```python
from build123d import *

# Parameters (mm, degrees)
F0_W     = 23.7
F0_H     = 15.8
F1_DEPTH = 10
F2_R     = 2.75
F3_DEPTH = 3
F4_W     = 20.786194
F4_H     = 12.840617
F5_DEPTH = 8
F6_R     = 3.802905
F6_R_2   = 2.49672
F6_R_3   = 2.479142
F7_DEPTH = 8


with BuildPart() as f1:
    # F0 (on Top) → F1 (new body)
    with BuildSketch(Plane.XY):
        with Locations((11.85, 7.9)):
            Rectangle(F0_W, F0_H)
    extrude(amount=F1_DEPTH)

    # F2 (on face) → F3 (join)
    with BuildSketch(Plane.XY.offset(10)):
        with Locations((4.25, 11.85)):
            Circle(F2_R)
        with Locations((11.75, 11.85)):
            Circle(F2_R)
        with Locations((19.25, 11.85)):
            Circle(F2_R)
        with Locations((4.25, 4.115675)):
            Circle(F2_R)
        with Locations((11.75, 4.115675)):
            Circle(F2_R)
        with Locations((19.25, 4.115675)):
            Circle(F2_R)
    extrude(amount=F3_DEPTH)

    # F4 (on face) → F5 (cut)
    with BuildSketch(Plane(origin=(0, 0, 0), x_dir=(1, 0, 0), z_dir=(0, 0, -1))):
        with Locations((11.888078, -7.852494)):
            Rectangle(F4_W, F4_H)
    extrude(amount=-F5_DEPTH, mode=Mode.SUBTRACT)

    # F6 (on face) → F7 (join)
    with BuildSketch(Plane(origin=(0, 0, 8), x_dir=(1, 0, 0), z_dir=(0, 0, -1))):
        with Locations((16.33504, -7.714347)):
            Circle(F6_R)
        with Locations((16.33504, -7.714347)):
            Circle(F6_R_2, mode=Mode.SUBTRACT)
        with Locations((6.87801, -7.714347)):
            Circle(F6_R)
        with Locations((6.87801, -7.714347)):
            Circle(F6_R_3, mode=Mode.SUBTRACT)
    extrude(amount=F7_DEPTH)


solid = f1.part
```
Here's how the part is built. I have some questions about the finished solid (model axes, mm). A direction names the side the tool comes from. Coordinates: 2 decimals unless noted, no trailing zeros. Order: outer loops, then holes, each group sorted by start corner. A loop starts at its lowest first (then second) coordinate and runs counter-clockwise, first axis right, second up. Notation, with made-up numbers: (-26, 18) - (22, 18) arc R35 cw to (22, 52) - close; hole circle Ø1 at (12, 30). An arc over 180 degrees is marked (long way). One line per question, with ' | ' between items. Start each with the question number.
1. If we section it at D-D (z = 10.75): Write out the boundary of the cut face in (x, y).
2. If we section it at A-A (z = 6.5): Write out the boundary of the cut face in (x, y).
3. Please list where these lines run through material, in increasing order: line 1 along Y through (x, z) = (4, 5.5); line 2 along Y through (x, z) = (11.25, 3.5); line 3 along X through (y, z) = (8, 1.5). Write a range as [from, to].
4. If we mould it in two halves opening along Y, with no side actions, what happens to faces 1 (the flat face through (19, 9, 0)), 2 (the cylindrical face through (18.09, 11.09, 4.06)), 3 (the flat face through (12, 15.8, 5))? For each: released by +Y, released by -Y, zero draft, split by the parting line, or undercut.
5. Which directions (+Z, -Z, +X, -X, +Y, -Y) give clear straight access to the entire face, cutting with the end or side of a thin tool? Please do faces 4 (the flat face through (4, 12, 13)), 5 (the cylindrical face through (5.5, 9.4, 11.5)), 6 (the cylindrical face through (13.84, 7.6, 4.06)).
6. If we section it at C-C (x = 11.75): Write out the boundary of the cut face in (y, z).
7. If we section it at B-B (y = 11.85): Write out the boundary of the cut face in (x, z).
Model answer:
1) outline: circle Ø5.5 at (4.25, 4.12); circle Ø5.5 at (4.25, 11.85); circle Ø5.5 at (11.75, 4.12); circle Ø5.5 at (11.75, 11.85); circle Ø5.5 at (19.25, 4.12); circle Ø5.5 at (19.25, 11.85)
2) outline: (0, 0) - (23.7, 0) - (23.7, 15.8) - (0, 15.8) - close; circle Ø7.61 at (6.88, 7.71); circle Ø7.61 at (16.34, 7.71); hole (1.49, 1.43) - (22.28, 1.43) - (22.28, 14.27) - (1.49, 14.27) - close; hole circle Ø4.96 at (6.88, 7.71); hole circle Ø4.99 at (16.34, 7.71)
3) line 1: y = [0, 1.43], [5.23, 10.2], [14.27, 15.8] | line 2: y = [0, 1.43], [14.27, 15.8] | line 3: x = [0, 1.49], [3.09, 4.42], [9.34, 10.67], [12.54, 13.85], [18.82, 20.13], [22.28, 23.7]
4) face 1: zero draft | face 2: undercut | face 3: released by +Y
5) face 4: +Z, +X, -X, +Y, -Y | face 5: +Z | face 6: -Z
6) outline: (0, 0) - (1.43, 0) - (1.43, 8) - (14.27, 8) - (14.27, 0) - (15.8, 0) - (15.8, 10) - (14.6, 10) - (14.6, 13) - (9.1, 13) - (9.1, 10) - (6.87, 10) - (6.87, 13) - (1.37, 13) - (1.37, 10) - (0, 10) - close
7) outline: (0, 0) - (1.49, 0) - (1.49, 8) - (22.28, 8) - (22.28, 0) - (23.7, 0) - (23.7, 10) - (22, 10) - (22, 13) - (16.5, 13) - (16.5, 10) - (14.5, 10) - (14.5, 13) - (9, 13) - (9, 10) - (7, 10) - (7, 13) - (1.5, 13) - (1.5, 10) - (0, 10) - close
